from build123d import *

# Parameters (mm, degrees)
SKETCH1_W           = 70
SKETCH1_H           = 50
BOSS_EXTRUDE1_DEPTH = 2
SKETCH2_R           = 1
BOSS_EXTRUDE2_DEPTH = 4
SKETCH3_R           = 2
BOSS_EXTRUDE3_DEPTH = 2
SKETCH4_W           = 62
SKETCH4_H           = 42
CUT_EXTRUDE1_DEPTH  = 2


with BuildPart() as part:
    # Sketch1 → Boss-Extrude1 (new body)
    with BuildSketch(Plane(origin=(0, 0, 0), x_dir=(1, 0, 0), z_dir=(0, 1, 0))):
        Rectangle(SKETCH1_W, SKETCH1_H)
    extrude(amount=BOSS_EXTRUDE1_DEPTH)

    # Sketch2 → Boss-Extrude2 (add)
    with BuildSketch(Plane(origin=(0, 2, 0), x_dir=(1, 0, 0), z_dir=(0, 1, 0))):
        with Locations(Location((-32.5, -23, 0), (0, 0, 90))):
            Circle(SKETCH2_R)
        with Locations(Location((-33, 23, 0), (0, 0, 90))):
            Circle(SKETCH2_R)
        with Locations(Location((32.5, 23, 0), (0, 0, 90))):
            Circle(SKETCH2_R)
        with Locations(Location((33, -23, 0), (0, 0, 90))):
            Circle(SKETCH2_R)
    extrude(amount=BOSS_EXTRUDE2_DEPTH)

    # Sketch3 → Boss-Extrude3 (add)
    with BuildSketch(Plane(origin=(0, 2, 0), x_dir=(1, 0, 0), z_dir=(0, 1, 0))):
        with Locations(Location((-33, 23, 0), (0, 0, 90))):
            Circle(SKETCH3_R)
        with Locations(Location((32.5, 23, 0), (0, 0, 90))):
            Circle(SKETCH3_R)
        with Locations(Location((33, -23, 0), (0, 0, 270))):
            Circle(SKETCH3_R)
        with Locations(Location((-32.5, -23, 0), (0, 0, 270))):
            Circle(SKETCH3_R)
    extrude(amount=BOSS_EXTRUDE3_DEPTH)

    # Sketch4 → Cut-Extrude1 (cut)
    with BuildSketch(Plane(origin=(0, 2, 0), x_dir=(1, 0, 0), z_dir=(0, 1, 0))):
        Rectangle(SKETCH4_W, SKETCH4_H)
    extrude(amount=-CUT_EXTRUDE1_DEPTH, mode=Mode.SUBTRACT)


solid = part.part
Geometry check sheet. Reference: the model listing, model coordinates, mm. A direction names the side the tool comes from. Give positions to 0.01 mm unless a question says otherwise; leave off trailing zeros. Loops run counter-clockwise (first coordinate to the right, second up) from the corner with the lowest first, then second, coordinate; pieces in that order, holes last. Notation, with made-up numbers: M 22,45.5 L 36,45.5 A26 cw 36,70.5 Z; hole C 88.5,38 d4. An arc over 180 degrees is marked long. Answer as a JSON object with one key per item and string values. Group by question number.
Item 1: Sectioned sample at A-A on x = 6.5. Record the boundary of the cut face in (y, z).
Item 2: Material ranges on L1, parallel to X at y = 1.3, z = 6.5; L2, parallel to Z at x = -26, y = 0.9; L3, parallel to X at y = 5.6, z = 22.5, recorded low to high.
Item 3: Mould release check, pull along X, two halves, no side actions. Record for faces 4 (the flat face through (-33, 6, 23)), 5 (the flat face through (0, 1, 21)), 6 (the flat face through (35, 1, 0)): pulls with the +X half, pulls with the -X half, needs draft (parallel to the pull), parting line crosses it, or undercut.
Item 4: Gauge pin test, flat ends, axial feed: pin 1 (1.5 mm diameter, centred on x = 0, y = 3, fed in from +Z); pin 2 (1 mm diameter, centred on x = -34, z = -24.5, fed in from +Y). Record the tip position at first contact, or that the pin passes through.
Item 5: Sectioned sample at C-C on y = 4.95. Record the boundary of the cut face in (x, z), plus the area to 3 significant figures.
Item 6: Access from +Z, -Z, +X, -X, +Y, -Y to the whole of each face (thin tool, end or side, straight path). Record for faces 1 (the flat face through (-5, 2, 22)), 2 (the flat face through (-31, 1, 0)), 3 (the flat face through (0, 1, 25)).
Item 7: Sectioned sample at B-B on z = 1. Record the boundary of the cut face in (x, y).
Findings below:
{
 "1": {"outline": "M 0,-25 L 2,-25 L 2,-21 L 0,-21 Z; M 0,21 L 2,21 L 2,25 L 0,25 Z"},
 "2": {"L1": "-35 to -31, 31 to 35", "L2": "-25 to -21, 21 to 25", "L3": "-33.37 to -31.63, 32.13 to 33.87"},
 "3": {"face 4": "needs draft", "face 5": "undercut", "face 6": "pulls with the +X half"},
 "4": {"pin 1": "through", "pin 2": "y = 4"},
 "5": {"outline": "C -33,-23 d2; C -32.5,23 d2; C 32.5,-23 d2; C 33,23 d2", "area": "12.6 mm2"},
 "6": {"face 1": "+Y", "face 2": "+Y, -Y", "face 3": "+Z, +X, -X, +Y, -Y"},
 "7": {"outline": "M -35,0 L -31,0 L -31,2 L -35,2 Z; M 31,0 L 35,0 L 35,2 L 31,2 Z"}
}
